Check sheet for the drawn part. Datum: minimum x, y, z corner. Units: mm. Round coordinates to 2 decimals unless told otherwise and drop trailing zeros. Order: outer loops, then holes, each group sorted by start corner. A loop starts at its lowest first (then second) coordinate and runs counter-clockwise, first axis right, second up.
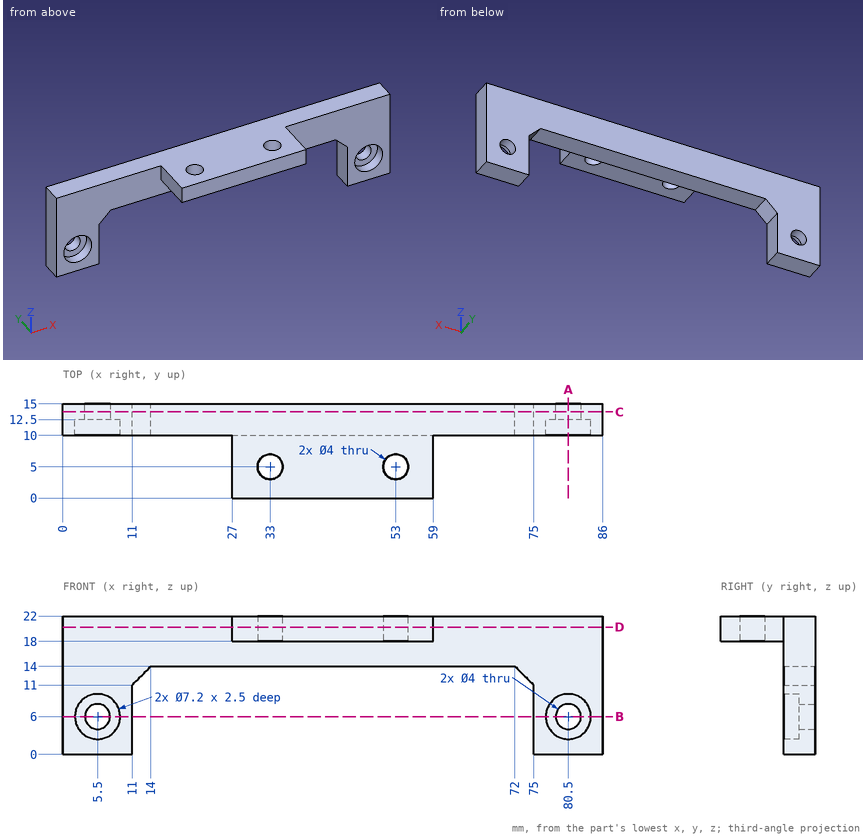
(1) Depth check by flat-ended pin: P1, Ø3, axis at y = 3, z = 19.5, coming from the +X side; P2, Ø1.5, axis at x = 36.5, y = 13, coming from the -Z side; P3, Ø5, axis at x = 47, y = 5, coming from the -Z side. Enter the tip coordinate at first touch or a pass-through.
Returned:
P1: stops at x = 59
P2: stops at z = 14
P3: stops at z = 18
(2) Sectioned sample at A-A, the plane x = 80.5. Record the cut outline in (y, z).
Returned:
outline: (10, 0) - (15, 0) - (15, 4) - (12.5, 4) - (12.5, 2.4) - (10, 2.4) - close; (10, 9.6) - (12.5, 9.6) - (12.5, 8) - (15, 8) - (15, 22) - (10, 22) - close
(3) Sectioned sample at C-C, the plane y = 13.75. Record the cut outline in (x, z).
Returned:
outline: (0, 0) - (11, 0) - (11, 11) - (14, 14) - (72, 14) - (75, 11) - (75, 0) - (86, 0) - (86, 22) - (0, 22) - close; hole circle Ø4 at (5.5, 6); hole circle Ø4 at (80.5, 6)
(4) Sectioned sample at B-B, the plane z = 6. Record the cut outline in (x, y), and give its area (3 significant figures).
Returned:
outline: (0, 10) - (1.9, 10) - (1.9, 12.5) - (3.5, 12.5) - (3.5, 15) - (0, 15) - close; (7.5, 12.5) - (9.1, 12.5) - (9.1, 10) - (11, 10) - (11, 15) - (7.5, 15) - close; (75, 10) - (76.9, 10) - (76.9, 12.5) - (78.5, 12.5) - (78.5, 15) - (75, 15) - close; (82.5, 12.5) - (84.1, 12.5) - (84.1, 10) - (86, 10) - (86, 15) - (82.5, 15) - close
area: 54.0 mm2
(5) Material ranges on line 1 (X direction, y = 5, z = 19.15); line 2 (X direction, y = 11.35, z = 6); line 3 (Z direction, x = 80.5, y = 13.5), recorded low to high.
Returned:
line 1: x = 27 to 31, 35 to 51, 55 to 59
line 2: x = 0 to 1.9, 9.1 to 11, 75 to 76.9, 84.1 to 86
line 3: z = 0 to 4, 8 to 22
(6) Sectioned sample at D-D, the plane z = 20.25. Record the cut outline in (x, y), and give its area (3 significant figures).
Returned:
outline: (0, 10) - (27, 10) - (27, 0) - (59, 0) - (59, 10) - (86, 10) - (86, 15) - (0, 15) - close; hole circle Ø4 at (33, 5); hole circle Ø4 at (53, 5)
area: 725 mm2
